from build123d import *

# Parameters (mm, degrees)
SKETCH1_W                  = 16
SKETCH1_H                  = 145
HOLE1_D                    = 180
HOLE1_CBORE_D              = 260
HOLE1_CBORE_DEPTH          = 4
F_8_4_8_4_DIAMETER_HOLE1_D = 8.4


with BuildPart() as part:
    # Sketch1 → Revolve1 (revolve)
    with BuildSketch(Plane(origin=(0, 0, 0), x_dir=(-1, 0, 0), z_dir=(0, 0, -1)), mode=Mode.PRIVATE) as revolve1_sk:
        with Locations((4, 72.5)):
            Rectangle(SKETCH1_W, SKETCH1_H)
    revolve(revolve1_sk.sketch.rotate(Axis((4, 0, 0), (-1, 0, 0)), 270), axis=Axis((4, 0, 0), (-1, 0, 0)))

    # Hole1 (through all)
    with Locations(Plane(origin=(4, 0, 0), x_dir=(0, 0, -1), z_dir=(1, 0, 0))):
        with Locations((0, 0)):
            CounterBoreHole(HOLE1_D / 2, HOLE1_CBORE_D / 2, HOLE1_CBORE_DEPTH)

    # Ø8.4 (8.4) Diameter Hole1 (through all)
    with Locations(Plane(origin=(0, 0, 0), x_dir=(0, 0, -1), z_dir=(1, 0, 0))):
        with Locations((110, 0), (95.262794416, 55), (55, 95.262794416), (0, 110), (-55, 95.262794416), (-95.262794416, 55), (-110, 0), (-95.262794416, -55), (-55, -95.262794416), (0, -110), (55, -95.262794416), (95.262794416, -55)):
            Hole(F_8_4_8_4_DIAMETER_HOLE1_D / 2)


solid = part.part
For this review, take the finished solid that the model builds, in its own axes (mm). A direction names the side the tool comes from. Round coordinates to 2 decimals unless told otherwise and drop trailing zeros. Loops run counter-clockwise (first coordinate to the right, second up) from the corner with the lowest first, then second, coordinate; pieces in that order, holes last. Notation, with made-up numbers: (-5.5, 31.5) - (9.5, 31.5) arc R31 ccw to (9.5, 61.5) - close; hole circle Ø10 at (54, 82). An arc over 180 degrees is marked (long way). Use one line per item in the form item = value.
1) Tool access review of faces 5 (the face through (0, 31, -85)), 6 (the face through (-6.084, -54.815, 91.067)): name each direction out of +Z, -Z, +X, -X, +Y, -Y from which nothing blocks a thin tool from reaching the whole face with its end or side.
Solutions:
face_5 = +X
face_6 = +X, -X
2) Clearance check with flat-ended pins moving along their axes: P1, Ø1, axis at x = 1, y = 64.5, coming from the -Z side; P2, Ø8, axis at x = -5, z = 105, coming from the +Y side; P3, Ø8, axis at x = -6.5, y = -33, coming from the -Z side. State where each tip first meets the part, or that it passes through.
Solutions:
P1 = -130.11
P2 = 104.04
P3 = -142.07
3) Mouldability with a two-part tool opening along Y and no side actions: class faces 1 (the face through (-6.08, 55.18, -99.46)), 2 (the face through (-6.084, -99.363, -55.91)), 3 (the face through (-12, 66, -62)), 4 (the face through (-4.112, 43.554, 138.304)) as pulls with the +Y half, pulls with the -Y half, needs draft (parallel to the pull), parting line crosses it, or undercut.
Solutions:
face_1 = undercut
face_2 = undercut
face_3 = needs draft
face_4 = parting line crosses it
4) Wall thickness on probe 1 along Y at (x, z) = (-6.25, 0); probe 2 along Z at (x, y) = (-1.25, 58); probe 3 along Y at (x, z) = (-4, -55): over which ranges is each line inside the solid? List them lowest first.
Solutions:
probe_1 = -145 to -114.2, -105.8 to -90, 90 to 105.8, 114.2 to 145
probe_2 = -132.89 to -98.2, -92.32 to -68.82, 68.82 to 92.32, 98.2 to 132.89
probe_3 = -134.16 to -99.46, -91.06 to -71.24, 71.24 to 91.06, 99.46 to 134.16
5) We need section D-D on y = 77. Write out the cut boundary in (x, z), then the cut area to 3 significant figures.
Solutions:
outline = (-12, -122.87) - (4, -122.87) - (4, -104.74) - (0, -104.74) - (0, -46.59) - (-12, -46.59) - close; (-12, 46.59) - (0, 46.59) - (0, 104.74) - (4, 104.74) - (4, 122.87) - (-12, 122.87) - close
area = 1,980 mm2
6) We need section A-A on y = 0. Write out the cut boundary in (x, z).
Solutions:
outline = (-12, -145) - (4, -145) - (4, -130) - (0, -130) - (0, -114.2) - (-12, -114.2) - close; (-12, -105.8) - (0, -105.8) - (0, -90) - (-12, -90) - close; (-12, 90) - (0, 90) - (0, 105.8) - (-12, 105.8) - close; (-12, 114.2) - (0, 114.2) - (0, 130) - (4, 130) - (4, 145) - (-12, 145) - close
7) We need section C-C on z = 110. Write out the cut boundary in (x, y), then the cut area to 3 significant figures.
Solutions:
outline = (-12, -94.47) - (4, -94.47) - (4, -69.28) - (0, -69.28) - (0, -4.2) - (-12, -4.2) - close; (-12, 4.2) - (0, 4.2) - (0, 69.28) - (4, 69.28) - (4, 94.47) - (-12, 94.47) - close
area = 2,370 mm2
